```python
from build123d import *

# Parameters (mm, degrees)
RESSALTO_EXTRUS_O4_DEPTH = 6
ESBO_O8_R                = 5.75
RESSALTO_EXTRUS_O7_DEPTH = 4
ESBO_O9_R                = 2.35
ESBO_O9_R_2              = 0.5
RESSALTO_EXTRUS_O8_DEPTH = 3
ESBO_O10_R               = 2.7
RESSALTO_EXTRUS_O9_DEPTH = 4
ESBO_O12_R               = 1
CORTE_EXTRUS_O1_DEPTH    = 25.203770367
FILETE1_R                = 1.5


with BuildPart() as part:
    # Esboço4 → Ressalto-extrusão4 (new, symmetric)
    with BuildSketch(Plane(origin=(0, 0, 0), x_dir=(1, 0, 0), z_dir=(0, 1, 0))):
        Polygon((-11.25, -10.5), (11.25, -10.5), (11.25, -6.5), (16.15, -6.5), (16.15, -4.5), (11.25, -4.5), (11.25, 10.5), (-11.25, 10.5), (-11.25, -4.5), (-16.15, -4.5), (-16.15, -6.5), (-11.25, -6.5), align=None)
    extrude(amount=RESSALTO_EXTRUS_O4_DEPTH, both=True)

    # Esboço8 → Ressalto-extrusão7 (add)
    with BuildSketch(Plane.XY.offset(10.5)):
        with Locations((5.5, 0)):
            Circle(ESBO_O8_R)
    extrude(amount=RESSALTO_EXTRUS_O7_DEPTH)

    # Esboço9 → Ressalto-extrusão8 (add)
    with BuildSketch(Plane.XY.offset(14.5)):
        with Locations((5.5, 0)):
            Circle(ESBO_O9_R)
        with Locations((5.5, 0)):
            Circle(ESBO_O9_R_2, mode=Mode.SUBTRACT)
    extrude(amount=RESSALTO_EXTRUS_O8_DEPTH)

    # Esboço10 → Ressalto-extrusão9 (add)
    with BuildSketch(Plane.XY.offset(10.5)):
        with Locations((-0.5, 0)):
            Circle(ESBO_O10_R)
    extrude(amount=RESSALTO_EXTRUS_O9_DEPTH)

    # Esboço12 → Corte-extrusão1 (cut, through all)
    with BuildSketch(Plane.XY.offset(6.5)):
        with Locations((-14, 0)):
            Circle(ESBO_O12_R)
        with Locations((14, 0)):
            Circle(ESBO_O12_R)
    extrude(amount=-CORTE_EXTRUS_O1_DEPTH, mode=Mode.SUBTRACT)

    # Filete1
    filete1_edges = [part.edges().sort_by_distance(p)[0] for p in [
        (16.15, -6, 5.5),
        (-16.15, -6, 5.5),
        (-16.15, 6, 5.5),
        (16.15, 6, 5.5),
    ]]
    fillet(filete1_edges, radius=FILETE1_R)


solid = part.part
```
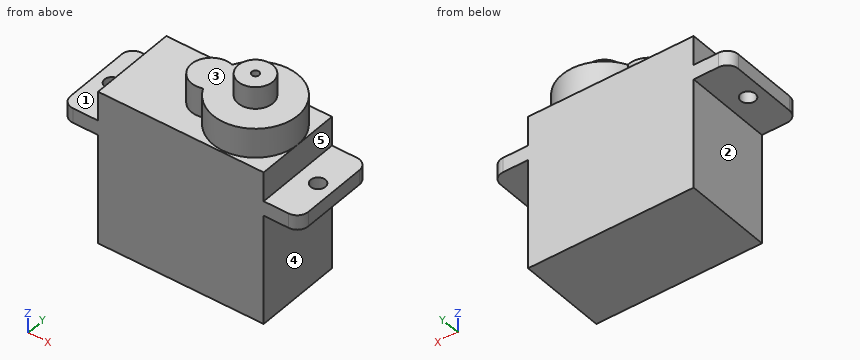
Input: part model. Units: mm. Frame: model coordinates. Face numbers are marked on the shaded views. A direction names the side the tool comes from. Give positions to 0.01 mm unless a question says otherwise; leave off trailing zeros. Order: outer loops, then holes, each group sorted by start corner. A loop starts at its lowest first (then second) coordinate and runs counter-clockwise, first axis right, second up. Notation, with made-up numbers: M 65.5,52.25 L 103.5,52.25 A31 ccw 103.5,85.25 Z; hole C 38,-29 d9. An arc over 180 degrees is marked long. Return JSON: item names as keys, results as strings.
1) Section query C-C on z = -3. Output: boundary loops of the cut face in (x, y), and give its area (3 significant figures).
Taken from the geometry:
{"outline": "M -11.25,-6 L 11.25,-6 L 11.25,6 L -11.25,6 Z", "area": "270 mm2"}
2) Line query: L1, parallel to Y at x = 14, z = 5; L2, parallel to Z at x = 15, y = 2.75; L3, parallel to Z at x = 2.5, y = -3.5. Output: solid intervals per line, ascending. Write a range as [from, to].
Taken from the geometry:
{"L1": "y = [-6, -1], [1, 6]", "L2": "z = [4.5, 6.5]", "L3": "z = [-10.5, 14.5]"}
3) Contact query for flat-ended pins moving along their axis: pin 1 (5 mm diameter, centred on y = -1.5, z = -6.5, fed in from +X); pin 2 (3.5 mm diameter, centred on x = 2, y = -0.5, fed in from +Z); pin 3 (4 mm diameter, centred on x = 14.5, y = 3, fed in from +Z); pin 4 (1.6 mm diameter, centred on x = 14, y = 0, fed in from -Z). Output: stop coordinate, or through.
Taken from the geometry:
{"pin 1": "stops at x = 11.25", "pin 2": "stops at z = 17.5", "pin 3": "stops at z = 6.5", "pin 4": "passes through"}
4) Access query for the marked faces 1, 2, 3, 4 and 5. Directions: +Z, -Z, +X, -X, +Y, -Y. A direction counts if a zero-diameter tool reaches every point of the face in a straight line with its end or side. Return the directions, or none.
Taken from the geometry:
{"face 1": "+Z, -X, +Y, -Y", "face 2": "-Z, -X, +Y, -Y", "face 3": "+Z", "face 4": "-Z, +X, +Y, -Y", "face 5": "+Z, +X, +Y, -Y"}
5) Section query B-B on x = -0.5. Output: boundary loops of the cut face in (y, z).
Taken from the geometry:
{"outline": "M -6,-10.5 L 6,-10.5 L 6,10.5 L 2.7,10.5 L 2.7,14.5 L -2.7,14.5 L -2.7,10.5 L -6,10.5 Z"}
6) Section query A-A on x = -14. Output: boundary loops of the cut face in (y, z).
Taken from the geometry:
{"outline": "M -6,4.5 L -1,4.5 L -1,6.5 L -6,6.5 Z; M 1,4.5 L 6,4.5 L 6,6.5 L 1,6.5 Z"}
7) Section query D-D on y = -1.5. Output: boundary loops of the cut face in (x, z) (3 decimals).
Taken from the geometry:
{"outline": "M -16.15,4.5 L -11.25,4.5 L -11.25,-10.5 L 11.25,-10.5 L 11.25,4.5 L 16.15,4.5 L 16.15,6.5 L 11.25,6.5 L 11.25,10.5 L 11.051,10.5 L 11.051,14.5 L 7.309,14.5 L 7.309,17.5 L 3.691,17.5 L 3.691,14.5 L -2.745,14.5 L -2.745,10.5 L -11.25,10.5 L -11.25,6.5 L -16.15,6.5 Z"}
